```python
from build123d import *

# Parameters (mm, degrees)
CYLINDER_R     = 1
CYLINDER_DEPTH = 10


with BuildPart() as cylinder:
    # Cylinder → Cylinder (new body)
    with BuildSketch(Plane.XY.offset(31)):
        Circle(CYLINDER_R)
    extrude(amount=CYLINDER_DEPTH)


with BuildPart() as obj1:
    # Cone → Cone (revolve)
    with BuildSketch(Plane.XZ):
        Polygon((0, 0), (2, 0), (4, 40), (0, 40), align=None)
    revolve(axis=Axis((0, 0, 0), (0, 0, 1)))

    # Cut003: cut Cylinder
    add(cylinder.part, mode=Mode.SUBTRACT)


with BuildPart() as obj1_1:
    # Cut003 placement: moved
    add(obj1.part.moved(Location((10, 25, -41.8))))


solid = obj1_1.part
```
Read the model definition and answer for the solid it produces. Units are mm, in the model's axes. A direction names the side the tool comes from. Round coordinates to 2 decimals unless told otherwise and drop trailing zeros. Write each loop counter-clockwise with the first axis right and the second up, starting at its lowest first coordinate (ties: lowest second). Pieces come first, ordered by that corner, then holes. Notation, with made-up numbers: (20, 45.25) - (40, 45.25) arc R21 ccw to (40, 66.25) - close; hole circle Ø5 at (7, 75). An arc over 180 degrees is marked (long way). One line per item, written item: value.
Q1. Straight lines are drawn through the part: line 1 (X direction, y = 25, z = -7); line 2 (Y direction, x = 10, z = -4.5) (3 decimals); line 3 (Y direction, x = 10, z = -8.5) (3 decimals). For each, find the intervals that lie inside material, in ascending order. Write a range as from..to.
The answers:
line 1: x = 6.26..9, 11..13.74
line 2: y = 21.135..24, 26..28.865
line 3: y = 21.335..24, 26..28.665
Q2. For a pull along Y with two mould halves and no side action, classify faces 3 (the flat face through (10, 25, -41.8)), 4 (the conical face through (11.391, 22.326, -21.52)), 5 (the cylindrical face through (10, 24, -6)) as pulls with the +Y half, pulls with the -Y half, needs draft (parallel to the pull), parting line crosses it, or undercut.
The answers:
face 3: needs draft
face 4: parting line crosses it
face 5: undercut
Q3. Find section C-C (z = -27). Determine the outline of the cut face in (x, y), and give its area (3 significant figures).
The answers:
outline: circle Ø5.48 at (10, 25)
area: 23.6 mm2
Q4. Each of these flat-tipped pins is pushed along its axis until it touches: P1, Ø3, axis at x = 12, z = -19.5, coming from the -Y side; P2, Ø3, axis at y = 25, z = -15, coming from the -X side (3 decimals); P3, Ø2, axis at y = 26, z = -12.5, coming from the -X side. Where does it stop, or does it pass through?
The answers:
P1: stops at y = 21.91
P2: stops at x = 6.585
P3: stops at x = 6.51
Q5. Find section B-B (y = 25). Determine the outline of the cut face in (x, z).
The answers:
outline: (6, -1.8) - (8, -41.8) - (12, -41.8) - (14, -1.8) - (11, -1.8) - (11, -10.8) - (9, -10.8) - (9, -1.8) - close
Q6. Find section A-A (x = 10). Determine the outline of the cut face in (y, z).
The answers:
outline: (21, -1.8) - (23, -41.8) - (27, -41.8) - (29, -1.8) - (26, -1.8) - (26, -10.8) - (24, -10.8) - (24, -1.8) - close
Q7. Find section D-D (z = -18). Determine the outline of the cut face in (x, y).
The answers:
outline: circle Ø6.38 at (10, 25)
Q8. Which of the six approach directions +Z, -Z, +X, -X, +Y, -Y give full straight-line access (tool end or side, diameter ignored) to faces 1 (the flat face through (10, 25, -10.8)), 2 (the flat face through (11, 24, -1.8))?
The answers:
face 1: +Z
face 2: +Z, +X, -X, +Y, -Y
